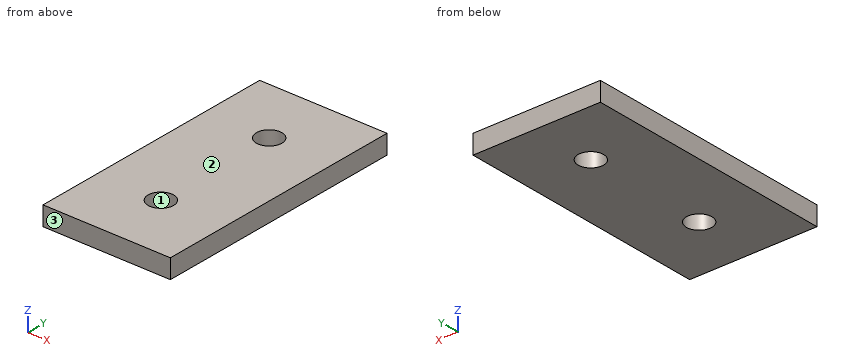
from build123d import *

# Parameters (mm, degrees)
SKETCH1_W           = 20
SKETCH1_H           = 40
BOSS_EXTRUDE1_DEPTH = 3
SKETCH2_R           = 2
CUT_EXTRUDE1_DEPTH  = 4
SKETCH3_R           = 2
CUT_EXTRUDE2_DEPTH  = 4


with BuildPart() as part:
    # Sketch1 → Boss-Extrude1 (new body)
    with BuildSketch(Plane.XY):
        with Locations((10, 20)):
            Rectangle(SKETCH1_W, SKETCH1_H)
    extrude(amount=BOSS_EXTRUDE1_DEPTH)

    # Sketch2 → Cut-Extrude1 (cut, through all)
    with BuildSketch(Plane.XY.offset(3)):
        with Locations((10, 10)):
            Circle(SKETCH2_R)
    extrude(amount=-CUT_EXTRUDE1_DEPTH, mode=Mode.SUBTRACT)

    # Sketch3 → Cut-Extrude2 (cut, through all)
    with BuildSketch(Plane.XY.offset(3)):
        with Locations((10, 30)):
            Circle(SKETCH3_R)
    extrude(amount=-CUT_EXTRUDE2_DEPTH, mode=Mode.SUBTRACT)


solid = part.part
Verification items for the finished model (mm, model axes). Face numbers are marked on the shaded views. Coordinates: 2 decimals unless noted, no trailing zeros. Loops run counter-clockwise (first coordinate to the right, second up) from the corner with the lowest first, then second, coordinate; pieces in that order, holes last. Notation, with made-up numbers: M 12.5,16 L 35.5,16 A10 cw 35.5,35 Z; hole C 50,33.5 d4. An arc over 180 degrees is marked long. One line per item, written item: value.
1. Mould release check, pull along Y, two halves, no side actions. Record for the marked faces 1, 2 and 3: pulls with the +Y half, pulls with the -Y half, needs draft (parallel to the pull), parting line crosses it, or undercut.
Answers follow:
face 1: undercut
face 2: needs draft
face 3: pulls with the -Y half
2. Section check A-A on y = 10. Record the cut outline in (x, z).
Answers follow:
outline: M 0,0 L 8,0 L 8,3 L 0,3 Z; M 12,0 L 20,0 L 20,3 L 12,3 Z
3. Section check C-C on z = 1.75. Record the cut outline in (x, y), plus the area to 3 significant figures.
Answers follow:
outline: M 0,0 L 20,0 L 20,40 L 0,40 Z; hole C 10,10 d4; hole C 10,30 d4
area: 775 mm^2
4. Section check D-D on y = 29. Record the cut outline in (x, z).
Answers follow:
outline: M 0,0 L 8.27,0 L 8.27,3 L 0,3 Z; M 11.73,0 L 20,0 L 20,3 L 11.73,3 Z
5. Section check B-B on x = 10. Record the cut outline in (y, z), plus the area to 3 significant figures.
Answers follow:
outline: M 0,0 L 8,0 L 8,3 L 0,3 Z; M 12,0 L 28,0 L 28,3 L 12,3 Z; M 32,0 L 40,0 L 40,3 L 32,3 Z
area: 96.0 mm^2
6. Material ranges on line 1 along Y through (x, z) = (10, 1.65); line 2 along Y through (x, z) = (8.25, 2.8), recorded low to high. Write a range as from..to.
Answers follow:
line 1: 0..8, 12..28, 32..40
line 2: 0..9.03, 10.97..29.03, 30.97..40
